Check sheet for the modelled part. Datum: model origin and axes. Units: mm. A direction names the side the tool comes from. Give positions to 0.01 mm unless a question says otherwise; leave off trailing zeros. Order: outer loops, then holes, each group sorted by start corner. A loop starts at its lowest first (then second) coordinate and runs counter-clockwise, first axis right, second up. Notation, with made-up numbers: (37, 12) -> (84, 12) arc R21 cw to (84, 40) -> close; hole circle Ø10 at (-38, 50.25). An arc over 180 degrees is marked (long way). Answer in a Markdown table with one row per item. Add a question column.
(1) Cross-section at C-C (y = 2.5). Record the cut outline in (x, z), then the cut area to 3 significant figures.
(2) Cross-section at A-A (x = 70). Record the cut outline in (y, z).
(3) Cross-section at B-B (z = -40.5). Record the cut outline in (x, y).
(4) Go/stop test with flat-tipped pins: pin 1 (0.6 mm diameter, centred on x = 48.5, y = 2.5, fed in from -Z); pin 2 (1 mm diameter, centred on y = 2.5, z = -15.5, fed in from +X); pin 3 (1 mm diameter, centred on y = 2, z = -3, fed in from +X). Record where each tip stops, or that it passes through.
(5) Thickness scan on L1, parallel to X at y = 0.25, z = -25; L2, parallel to Z at x = 22.5, y = 0.45; L3, parallel to X at y = 2.35, z = -2.5. Record the ranges inside material, lowest first. Write a range as [from, to].
(6) Set-up check for faces 5 (the face through (43, 2, -44.2)), 6 (the face through (19.04, 0.3, -18.21)), 7 (the face through (2.01, 1.8, -46.4)): record each of +Z, -Z, +X, -X, +Y, -Y from which the full face is reachable in a straight line by a thin tool's end or side.
(7) Release check for a two-part mould opening along Y. For faces 1 (the face through (2.01, 2, -3)), 2 (the face through (0.99, 2.27, -2.11)), 3 (the face through (0, 2, -24)), 4 (the face through (43.47, 2.2, -46.07)) record: released by +Y, released by -Y, zero draft, split by the parting line, or undercut.
(8) Cross-section at D-D (z = -31). Record the cut outline in (x, y), then the cut area to 3 significant figures.
```python
from build123d import *

# Parameters (mm, degrees)
ESBO_O1_W                = 85.8
ESBO_O1_H                = 49.2
RESSALTO_EXTRUS_O1_DEPTH = 1.26
RESSALTO_EXTRUS_O5_DEPTH = 2.01
RESSALTO_EXTRUS_O6_REACH = 102.969
RESSALTO_EXTRUS_O6_START = -2.01
CORTE_EXTRUS_O4_DEPTH    = 0.6


with BuildPart() as part:
    # Esboço1 → Ressalto-extrusão1 (new body)
    with BuildSketch(Plane(origin=(0, 0, 0), x_dir=(1, 0, 0), z_dir=(0, 1, 0))):
        with Locations((42.9, 24.6)):
            Rectangle(ESBO_O1_W, ESBO_O1_H)
    extrude(amount=RESSALTO_EXTRUS_O1_DEPTH)

    # Esboço9 → Ressalto-extrusão5 (add)
    with BuildSketch(Plane.ZY):
        Polygon((-47.19, 1.26), (-46.989750156, 3.26), (-2.210249844, 3.26), (-2.01, 1.26), align=None)
    extrude(amount=-RESSALTO_EXTRUS_O5_DEPTH)

    # Esboço11 → Ressalto-extrusão6 (add, up to next)
    with BuildSketch(Plane(origin=(85.8, 0, 0), x_dir=(0, 0, -1), z_dir=(1, 0, 0)).offset(RESSALTO_EXTRUS_O6_START), mode=Mode.PRIVATE) as ressalto_extrus_o6_sk1:
        Polygon((44.2, 1.26), (45.2, 1.26), (46.959846557, 3.16027369), (46.952453114, 3.26), (44.2, 3.26), align=None)
    ressalto_extrus_o6_tool1 = extrude(ressalto_extrus_o6_sk1.sketch, amount=-RESSALTO_EXTRUS_O6_REACH, mode=Mode.PRIVATE) - part.part
    # Esboço11 → Ressalto-extrusão6 (add, up to next)
    with BuildSketch(Plane(origin=(85.8, 0, 0), x_dir=(0, 0, -1), z_dir=(1, 0, 0)).offset(RESSALTO_EXTRUS_O6_START), mode=Mode.PRIVATE) as ressalto_extrus_o6_sk2:
        Polygon((5, 3.26), (5, 1.26), (4, 1.26), (2.240153443, 3.16027369), (2.247546886, 3.26), align=None)
    ressalto_extrus_o6_tool2 = extrude(ressalto_extrus_o6_sk2.sketch, amount=-RESSALTO_EXTRUS_O6_REACH, mode=Mode.PRIVATE) - part.part
    add(ressalto_extrus_o6_tool1.solids().sort_by_distance((83.79, 2.41923, -45.235001))[0])
    add(ressalto_extrus_o6_tool2.solids().sort_by_distance((83.79, 2.41923, -3.964999))[0])

    # Esboço8 → Corte-extrusão4 (cut)
    with BuildSketch(Plane.XZ):
        with BuildLine():
            ThreePointArc((22.054636183, -24.574784692), (19.006183567, -30.839043664), (24.543756305, -35.066252199))
            ThreePointArc((24.543756305, -35.066252199), (34.411504106, -32.18495748), (41.324551108, -24.576798237))
            ThreePointArc((41.324551108, -24.576798237), (34.411504106, -16.968638994), (24.543756305, -14.087344275))
            ThreePointArc((24.543756305, -14.087344275), (19.015675216, -18.314400935), (22.054636183, -24.574784692))
        make_face()
        with BuildLine():
            ThreePointArc((24.533243249, -14.587267716), (19.371981333, -19.36170914), (24.08768254, -24.576695007))
            ThreePointArc((24.08768254, -24.576695007), (19.36258934, -29.791975707), (24.532809194, -34.566332751))
            ThreePointArc((24.532809194, -34.566332751), (34.03743393, -31.828610978), (40.763816601, -24.576798237))
            ThreePointArc((40.763816601, -24.576798237), (34.037618764, -17.325099255), (24.533243249, -14.587267716))
        make_face(mode=Mode.SUBTRACT)
    extrude(amount=-CORTE_EXTRUS_O4_DEPTH, mode=Mode.SUBTRACT)


solid = part.part
```
Answer below:
| question | item | result |
|---|---|---|
| 1 | outline | (0, -47.07) -> (2.01, -47.07) -> (2.01, -46.35) -> (83.79, -46.35) -> (83.79, -44.2) -> (2.01, -44.2) -> (2.01, -5) -> (83.79, -5) -> (83.79, -2.85) -> (2.01, -2.85) -> (2.01, -2.13) -> (0, -2.13) -> close |
| 1 | area | 442 mm² |
| 2 | outline | (0, -49.2) -> (1.26, -49.2) -> (1.26, -45.2) -> (3.16, -46.96) -> (3.26, -46.95) -> (3.26, -44.2) -> (1.26, -44.2) -> (1.26, -5) -> (3.26, -5) -> (3.26, -2.25) -> (3.16, -2.24) -> (1.26, -4) -> (1.26, 0) -> (0, 0) -> close |
| 3 | outline | (0, 0) -> (85.8, 0) -> (85.8, 1.26) -> (2.01, 1.26) -> (2.01, 3.26) -> (0, 3.26) -> close |
| 4 | pin 1 | stops at z = -46.63 |
| 4 | pin 2 | stops at x = 2.01 |
| 4 | pin 3 | stops at x = 83.79 |
| 5 | L1 | x = [0, 21.3], [22.33, 40.54], [41.11, 85.8] |
| 5 | L2 | z = [-49.2, -34.75], [-34.21, -24.93], [-24.22, -14.95], [-14.41, 0] |
| 5 | L3 | x = [0, 2.01] |
| 6 | face 5 | +X, +Y |
| 6 | face 6 | -Y |
| 6 | face 7 | -Z, +X |
| 7 | face 1 | undercut |
| 7 | face 2 | released by +Y |
| 7 | face 3 | zero draft |
| 7 | face 4 | undercut |
| 8 | outline | (0, 0) -> (19.05, 0) -> (19.05, 0.6) -> (19.57, 0.6) -> (19.57, 0) -> (35.27, 0) -> (35.27, 0.6) -> (36.1, 0.6) -> (36.1, 0) -> (85.8, 0) -> (85.8, 1.26) -> (2.01, 1.26) -> (2.01, 3.26) -> (0, 3.26) -> close |
| 8 | area | 111 mm² |
